Design review of the part built by this model. Coordinates are the model's own, in mm. A direction names the side the tool comes from. Coordinates: 2 decimals unless noted, no trailing zeros. Write each loop counter-clockwise with the first axis right and the second up, starting at its lowest first coordinate (ties: lowest second). Pieces come first, ordered by that corner, then holes. Notation, with made-up numbers: M -7.5,19.5 L 2.5,19.5 A14 cw 2.5,36.5 Z; hole C 37,3.25 d2. An arc over 180 degrees is marked long. Write item = value, one per line.
```python
from build123d import *

# Parameters (mm, degrees)
F0_W           = 128.778
F0_H           = 125.476
F1_DEPTH       = 673.1
F2_W           = 88.9
F2_H           = 88.9
F3_DEPTH       = 508
F4_W           = 141.477994
F4_H           = 138.175994
F4_W_2         = 88.9
F4_H_2         = 88.9
F5_DEPTH       = 12.7
F6_W           = 141.477994
F6_H           = 138.175994
F6_W_2         = 128.778
F6_H_2         = 125.476
F7_DEPTH       = 6.35
F8_W           = 38.1
F8_H           = 38.1
F9_DEPTH       = 495.3
F10_W          = 139.7
F10_H          = 139.7
F10_W_2        = 127
F10_H_2        = 127
F11_DEPTH      = 6.35
F12_W          = 139.7
F12_H          = 139.7
F13_DEPTH      = 12.7
F14_W          = 50.8
F14_H          = 127
F15_DEPTH      = 25.4
F15_DEPTH_BACK = 114.3
F16_W          = 50.8
F16_H          = 127
F17_DEPTH      = 25.4
F17_DEPTH_BACK = 114.3
F18_W          = 127
F18_H          = 127
F19_DEPTH      = 19.05


with BuildPart() as f1:
    # F0 (on Top) → F1 (new body)
    with BuildSketch(Plane.XY):
        Rectangle(F0_W, F0_H)
    extrude(amount=F1_DEPTH)

    # F2 (on face) → F3 (join)
    with BuildSketch(Plane.XY.offset(673.1)):
        Rectangle(F2_W, F2_H)
    extrude(amount=F3_DEPTH)

    # F4 (on face) → F5 (join)
    with BuildSketch(Plane.XY.offset(673.1)):
        Rectangle(F4_W, F4_H)
        Rectangle(F4_W_2, F4_H_2, mode=Mode.SUBTRACT)
    extrude(amount=F5_DEPTH)

    # F6 (on face) → F7 (join)
    with BuildSketch(Plane(origin=(0, 0, 673.1), x_dir=(1, 0, 0), z_dir=(0, 0, -1))):
        Rectangle(F6_W, F6_H)
        Rectangle(F6_W_2, F6_H_2, mode=Mode.SUBTRACT)
    extrude(amount=F7_DEPTH)

    # F8 (on face) → F9 (join)
    with BuildSketch(Plane.XY.offset(685.8)):
        with Locations((44.45, 44.45)):
            Rectangle(F8_W, F8_H)
        with Locations((44.45, -44.45)):
            Rectangle(F8_W, F8_H)
        with Locations((-44.45, -44.45)):
            Rectangle(F8_W, F8_H)
        with Locations((-44.45, 44.45)):
            Rectangle(F8_W, F8_H)
    extrude(amount=F9_DEPTH)

    # F10 (on face) → F11 (join)
    with BuildSketch(Plane.XY.offset(1181.1)):
        Rectangle(F10_W, F10_H)
        Rectangle(F10_W_2, F10_H_2, mode=Mode.SUBTRACT)
    extrude(amount=-F11_DEPTH)

    # F12 (on face) → F13 (join)
    with BuildSketch(Plane.XY.offset(1181.1)):
        Rectangle(F12_W, F12_H)
    extrude(amount=F13_DEPTH)

    # F14 (on face) → F15 (join, two sides)
    with BuildSketch(Plane.XZ.offset(44.45)) as f15_sk:
        with Locations((0, 1060.45)):
            Rectangle(F14_W, F14_H)
    extrude(amount=F15_DEPTH)
    extrude(f15_sk.sketch, amount=-F15_DEPTH_BACK)

    # F16 (on face) → F17 (join, two sides)
    with BuildSketch(Plane.YZ.offset(44.45)) as f17_sk:
        with Locations((0, 1060.45)):
            Rectangle(F16_W, F16_H)
    extrude(amount=F17_DEPTH)
    extrude(f17_sk.sketch, amount=-F17_DEPTH_BACK)

    # F18 (on face) → F19 (join)
    with BuildSketch(Plane.XY.offset(1193.8)):
        Rectangle(F18_W, F18_H)
    extrude(amount=F19_DEPTH)


solid = f1.part
```
Q1. For P1, Ø1, axis at y = 46.5, z = 1032.5, coming from the +X side; P2, Ø1.9, axis at y = -65, z = 1077.5, coming from the -X side; P3, Ø21, axis at y = -1, z = 1187.5, coming from the +X side, all flat-tipped, find the tip position at first contact; note any pin that passes through.
Check result:
P1 = 63.5
P2 = -25.4
P3 = 69.85
Q2. Wall thickness on line 1 (Z direction, x = -44.5, y = -16); line 2 (Y direction, x = 45, z = 910); line 3 (Z direction, x = -57, y = -64): over which ranges is each line inside the solid? List them lowest first.
Check result:
line_1 = 0 to 685.8, 996.95 to 1123.95, 1181.1 to 1212.85
line_2 = -63.5 to -25.4, 25.4 to 63.5
line_3 = 666.75 to 685.8, 1174.75 to 1193.8
Q3. Consider section D-D, the plane z = 830.5. State the section outline as (x, y) points, and give its area (3 significant figures).
Check result:
outline = M -63.5,-63.5 L -25.4,-63.5 L -25.4,-44.45 L 25.4,-44.45 L 25.4,-63.5 L 63.5,-63.5 L 63.5,-25.4 L 44.45,-25.4 L 44.45,25.4 L 63.5,25.4 L 63.5,63.5 L 25.4,63.5 L 25.4,44.45 L -25.4,44.45 L -25.4,63.5 L -63.5,63.5 L -63.5,25.4 L -44.45,25.4 L -44.45,-25.4 L -63.5,-25.4 Z
area = 12,300 mm²
Q4. Consider section B-B, the plane z = 1085.5. State the section outline as (x, y) points.
Check result:
outline = M -69.85,-25.4 L -63.5,-25.4 L -63.5,-63.5 L -25.4,-63.5 L -25.4,-69.85 L 25.4,-69.85 L 25.4,-63.5 L 63.5,-63.5 L 63.5,-25.4 L 69.85,-25.4 L 69.85,25.4 L 63.5,25.4 L 63.5,63.5 L 25.4,63.5 L 25.4,69.85 L -25.4,69.85 L -25.4,63.5 L -63.5,63.5 L -63.5,25.4 L -69.85,25.4 Z
Q5. Machinability: for faces 1 (the flat face through (-1, -62.738, 329)), 2 (the flat face through (-63.5, -45, 927)), 3 (the flat face through (63.5, -45, 927)), which of the approach directions +Z, -Z, +X, -X, +Y, -Y give a long, thin tool a straight path to every point of the face, cutting with its end or side? Answer none if there is none.
Check result:
face_1 = -Z, +X, -X, -Y
face_2 = -X, -Y
face_3 = +X, -Y
Q6. The part is to be moulded in two halves that separate along X. For faces 4 (the flat face through (-1, 1, 1212.85)), 5 (the flat face through (63.5, -1, 1203)), 6 (the flat face through (-25.4, 54, 1152)), say which applies: +X half, -X half, draft (parallel to the pull), parting line (faces both ways), or undercut.
Check result:
face_4 = draft
face_5 = +X half
face_6 = undercut
